Build history of the part. All positions in model axes, mm. Give positions to 0.01 mm unless a question says otherwise; leave off trailing zeros. Loops run counter-clockwise (first coordinate to the right, second up) from the corner with the lowest first, then second, coordinate; pieces in that order, holes last. Notation, with made-up numbers: M 56,-1 L 83,-1 A30 ccw 83,34 Z; hole C 47,73.25 d9. An arc over 180 degrees is marked long. Answer in a Markdown table with one row per item. Add a question column.
```python
from build123d import *

# Parameters (mm, degrees)
SKETCH1_W                   = 19.05
SKETCH1_H                   = 19.05
BOSS_EXTRUDE1_DEPTH         = 25.4
TAP_DRILL_FOR_M4X0_7_TAP1_D = 3.3
M8_CLEARANCE_HOLE1_D        = 9


with BuildPart() as part:
    # Sketch1 → Boss-Extrude1 (new, symmetric)
    with BuildSketch(Plane.XY):
        Rectangle(SKETCH1_W, SKETCH1_H)
    extrude(amount=BOSS_EXTRUDE1_DEPTH, both=True)

    # Tap Drill for M4x0.7 Tap1 (through all)
    with Locations(Plane(origin=(0, 9.525, 0), x_dir=(1, 0, 0), z_dir=(0, 1, 0))):
        with Locations((0, 20), (0, -20)):
            Hole(TAP_DRILL_FOR_M4X0_7_TAP1_D / 2)

    # M8 Clearance Hole1 (through all)
    with Locations(Plane.ZY.offset(9.525)):
        with Locations((0, -0.975)):
            Hole(M8_CLEARANCE_HOLE1_D / 2)


solid = part.part
```
(1) Slice it at D-D, the plane z = 0. Give the cut face in (x, y) (3 decimals).
(2) Pull direction Z, two halves, no side cores. Call faces 1 (the flat face through (0, 0, 25.4)), 2 (the flat face through (9.525, 4, 0)), 3 (the flat face through (0, 0, -25.4)), 4 (the cylindrical face through (0.215, -0.133, 18.364)): +Z half, -Z half, draft (parallel to the pull), parting line (faces both ways), or undercut.
(3) Slice it at B-B, the plane x = 0. Give the cut face in (y, z) (3 decimals).
(4) Slice it at C-C, the plane y = 0.25. Give the cut face in (x, z) (3 decimals), then the cut area to 3 significant figures.
(5) Wall check: line 1 (X direction, y = -4.75, z = -20) (3 decimals); line 2 (Z direction, x = -1.5, y = 0.75); line 3 (Z direction, x = 0, y = -4.25). Give the ranges that are in metal, low to high.
(6) Slice it at A-A, the plane z = 20. Give the cut face in (x, y) (3 decimals).
(7) Pin check, flat tips, straight feed: pin 1 (5 mm diameter, centred on y = -2, z = 2, fed in from -X) (3 decimals); pin 2 (2 mm diameter, centred on x = 0, z = -20, fed in from +Y). Stop position of each tip, or through.
Solution:
| question | item | result |
|---|---|---|
| 1 | outline | M -9.525,-9.525 L 9.525,-9.525 L 9.525,-5.475 L -9.525,-5.475 Z; M -9.525,3.525 L 9.525,3.525 L 9.525,9.525 L -9.525,9.525 Z |
| 2 | face 1 | +Z half |
| 2 | face 2 | draft |
| 2 | face 3 | -Z half |
| 2 | face 4 | undercut |
| 3 | outline | M -9.525,-25.4 L 9.525,-25.4 L 9.525,-21.65 L -9.525,-21.65 Z; M -9.525,-18.35 L 9.525,-18.35 L 9.525,18.35 L -9.525,18.35 Z; M -9.525,21.65 L 9.525,21.65 L 9.525,25.4 L -9.525,25.4 Z; hole C -0.975,0 d9 |
| 4 | outline | M -9.525,-25.4 L 9.525,-25.4 L 9.525,-4.33 L -9.525,-4.33 Z; M -9.525,4.33 L 9.525,4.33 L 9.525,25.4 L -9.525,25.4 Z; hole C 0,-20 d3.3; hole C 0,20 d3.3 |
| 4 | area | 786 mm^2 |
| 5 | line 1 | -9.525 to -1.65, 1.65 to 9.525 |
| 5 | line 2 | -25.4 to -20.69, -19.31 to -4.16, 4.16 to 19.31, 20.69 to 25.4 |
| 5 | line 3 | -25.4 to -21.65, -18.35 to -3.09, 3.09 to 18.35, 21.65 to 25.4 |
| 6 | outline | M -9.525,-9.525 L -1.65,-9.525 L -1.65,9.525 L -9.525,9.525 Z; M 1.65,-9.525 L 9.525,-9.525 L 9.525,9.525 L 1.65,9.525 Z |
| 7 | pin 1 | x = -9.525 |
| 7 | pin 2 | through |
